from build123d import *

# Parameters (mm, degrees)
F0_W     = 70
F0_H     = 65
F1_DEPTH = 25
F2_W     = 40
F2_H     = 50
F3_DEPTH = 20
F5_DEPTH = 25.001
F7_DEPTH = 25.001
F8_R     = 2
F8_R_2   = 1.75
F9_DEPTH = 25.001


with BuildPart() as f1:
    # F0 (on Front) → F1 (new body)
    with BuildSketch(Plane.XZ):
        Rectangle(F0_W, F0_H)
    extrude(amount=F1_DEPTH)

    # F2 (on face) → F3 (cut)
    with BuildSketch(Plane.XZ.offset(25)):
        Rectangle(F2_W, F2_H)
    extrude(amount=-F3_DEPTH, mode=Mode.SUBTRACT)

    # F4 (on face) → F5 (cut, through all)
    with BuildSketch(Plane.XZ.offset(25)):
        with BuildLine():
            Line((-35, 22.5), (-35, -32.5))
            Line((-35, -32.5), (-27.5, -32.5))
            Line((-27.5, -32.5), (-27.5, 20.5))
            ThreePointArc((-27.5, 20.5), (-28.085786, 21.914214), (-29.5, 22.5))
            Line((-29.5, 22.5), (-35, 22.5))
        make_face()
    extrude(amount=-F5_DEPTH, mode=Mode.SUBTRACT)

    # F6 (on face) → F7 (cut, through all)
    with BuildSketch(Plane.XZ.offset(25)):
        with BuildLine():
            Line((35, -22.5), (35, 32.5))
            Line((35, 32.5), (27.5, 32.5))
            Line((27.5, 32.5), (27.5, -20.5))
            ThreePointArc((27.5, -20.5), (28.085786, -21.914214), (29.5, -22.5))
            Line((29.5, -22.5), (35, -22.5))
        make_face()
    extrude(amount=-F7_DEPTH, mode=Mode.SUBTRACT)

    # F8 (on face) → F9 (cut, through all)
    with BuildSketch(Plane.XZ.offset(25)):
        with Locations((-31, 27.5)):
            Circle(F8_R)
        with Locations((31, -27.5)):
            Circle(F8_R)
        with Locations((-23, 28.5)):
            Circle(F8_R_2)
        with Locations((23, 28.5)):
            Circle(F8_R_2)
        with Locations((-23, -28.5)):
            Circle(F8_R_2)
        with Locations((23, -28.5)):
            Circle(F8_R_2)
    extrude(amount=-F9_DEPTH, mode=Mode.SUBTRACT)


solid = f1.part
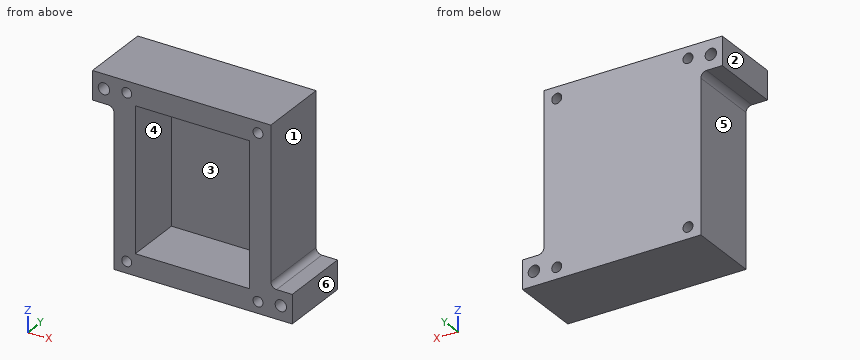
Design review of the part built by this model. Coordinates are the model's own, in mm. Face numbers are marked on the shaded views. A direction names the side the tool comes from. Round coordinates to 2 decimals unless told otherwise and drop trailing zeros. Write each loop counter-clockwise with the first axis right and the second up, starting at its lowest first coordinate (ties: lowest second). Pieces come first, ordered by that corner, then holes. Notation, with made-up numbers: (-34, -40) -> (13, -40) arc R19 ccw to (13, -19) -> close; hole circle Ø3 at (-23.5, 66.5). An arc over 180 degrees is marked (long way). One line per question, with ' | ' between items.
(1) Take a section at C-C, the plane z = 9. State the section outline as (x, y) points.
Result sheet:
outline: (-27.5, -25) -> (-20, -25) -> (-20, -5) -> (20, -5) -> (20, -25) -> (27.5, -25) -> (27.5, 0) -> (-27.5, 0) -> close
(2) Take a section at A-A, the plane y = -14. State the section outline as (x, z) points, and give its area (3 significant figures).
Result sheet:
outline: (-35, 22.5) -> (-29.5, 22.5) arc R2 cw to (-27.5, 20.5) -> (-27.5, -32.5) -> (35, -32.5) -> (35, -22.5) -> (29.5, -22.5) arc R2 cw to (27.5, -20.5) -> (27.5, 32.5) -> (-35, 32.5) -> close; hole circle Ø4 at (-31, 27.5); hole circle Ø3.5 at (-23, -28.5); hole circle Ø3.5 at (-23, 28.5); hole (-20, -25) -> (20, -25) -> (20, 25) -> (-20, 25) -> close; hole circle Ø3.5 at (23, -28.5); hole circle Ø3.5 at (23, 28.5); hole circle Ø4 at (31, -27.5) | area: 1,660 mm2
(3) Machinability: for the marked faces 4, 5 and 6, which of the approach directions +Z, -Z, +X, -X, +Y, -Y give a long, thin tool a straight path to every point of the face, cutting with its end or side? Answer none if there is none.
Result sheet:
face 4: -Y | face 5: -Z, -X, +Y, -Y | face 6: +Z, -Z, +X, +Y, -Y
(4) Take a section at B-B, the plane x = 31. State the section outline as (y, z) points, and give its area (3 significant figures).
Result sheet:
outline: (-25, -32.5) -> (0, -32.5) -> (0, -29.5) -> (-25, -29.5) -> close; (-25, -25.5) -> (0, -25.5) -> (0, -22.5) -> (-25, -22.5) -> close | area: 150 mm2
(5) Take a section at D-D, the plane x = -23. State the section outline as (y, z) points.
Result sheet:
outline: (-25, -32.5) -> (0, -32.5) -> (0, -30.25) -> (-25, -30.25) -> close; (-25, -26.75) -> (0, -26.75) -> (0, 26.75) -> (-25, 26.75) -> close; (-25, 30.25) -> (0, 30.25) -> (0, 32.5) -> (-25, 32.5) -> close
(6) Wall thickness on line 1 (Z direction, x = 23, y = -17.25); line 2 (X direction, y = -15.5, z = -15); line 3 (Z direction, x = 12, y = -21.5): over which ranges is each line inside the solid? List them lowest first. Write a range as [from, to].
Result sheet:
line 1: [-32.5, -30.25], [-26.75, 26.75], [30.25, 32.5] | line 2: [-27.5, -20], [20, 27.5] | line 3: [-32.5, -25], [25, 32.5]
(7) Draft analysis for pull direction X (two halves, no side actions). For the marked faces 1, 2 and 3, state which applies: released by +X, released by -X, zero draft, split by the parting line, or undercut.
Result sheet:
face 1: released by +X | face 2: released by -X | face 3: undercut
(8) Insertion check: P1, Ø7.5, axis at y = -16, z = 6, coming from the -X side; P2, Ø2, axis at y = -10, z = 10, coming from the +X side; P3, Ø12, axis at x = 6.5, z = -9, coming from the -Y side. Each pin has a flat end and moves straight along its axis. Give the tip position at first contact, or say it passes through.
Result sheet:
P1: x = -27.5 | P2: x = 27.5 | P3: y = -5
